Check sheet for the drawn part. Datum: minimum x, y, z corner. Units: mm. Give positions to 0.01 mm unless a question says otherwise; leave off trailing zeros. Order: outer loops, then holes, each group sorted by start corner. A loop starts at its lowest first (then second) coordinate and runs counter-clockwise, first axis right, second up.
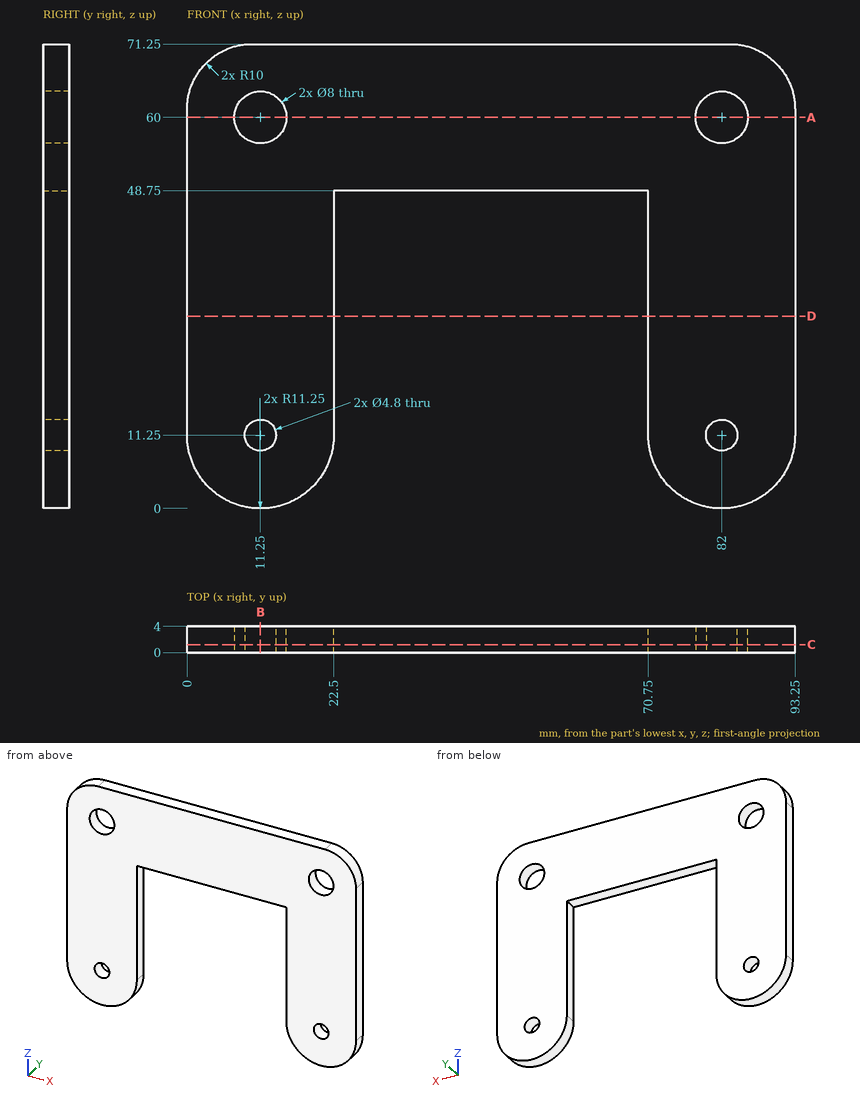
Item 1: Scan lines: L1, parallel to X at y = 3.15, z = 60; L2, parallel to Z at x = 82, y = 3.1; L3, parallel to X at y = 3.25, z = 24.5. Record each from-to range of solid material in increasing order.
Reported:
L1: x = 0 to 7.25, 15.25 to 78, 86 to 93.25
L2: z = 0 to 8.85, 13.65 to 56, 64 to 71.25
L3: x = 0 to 22.5, 70.75 to 93.25
Item 2: Sectioned sample at C-C (y = 1.2). Enter the section's corners in (x, z).
Reported:
outline: (0, 11.25) arc R11.25 ccw to (22.5, 11.25) - (22.5, 48.75) - (70.75, 48.75) - (70.75, 11.25) arc R11.25 ccw to (93.25, 11.25) - (93.25, 61.25) arc R10 ccw to (83.25, 71.25) - (10, 71.25) arc R10 ccw to (0, 61.25) - close; hole circle Ø8 at (11.25, 60); hole circle Ø4.8 at (11.25, 11.25); hole circle Ø8 at (82, 60); hole circle Ø4.8 at (82, 11.25)
Item 3: Sectioned sample at A-A (z = 60). Enter the section's corners in (x, y), and give its area (3 significant figures).
Reported:
outline: (0, 0) - (7.25, 0) - (7.25, 4) - (0, 4) - close; (15.25, 0) - (78, 0) - (78, 4) - (15.25, 4) - close; (86, 0) - (93.25, 0) - (93.25, 4) - (86, 4) - close
area: 309 mm2
Item 4: Gauge pin test, flat end, axial feed: pin 1 (2 mm diameter, centred on x = 47.5, y = 2, fed in from -Z). Record the tip position at first contact, or that the pin passes through.
Reported:
pin 1: stops at z = 48.75
Item 5: Sectioned sample at D-D (z = 29.5). Enter the section's corners in (x, y), and give its area (3 significant figures).
Reported:
outline: (0, 0) - (22.5, 0) - (22.5, 4) - (0, 4) - close; (70.75, 0) - (93.25, 0) - (93.25, 4) - (70.75, 4) - close
area: 180 mm2
Item 6: Sectioned sample at B-B (x = 11.25). Enter the section's corners in (y, z), and give its area (3 significant figures).
Reported:
outline: (0, 0) - (4, 0) - (4, 8.85) - (0, 8.85) - close; (0, 13.65) - (4, 13.65) - (4, 56) - (0, 56) - close; (0, 64) - (4, 64) - (4, 71.25) - (0, 71.25) - close
area: 234 mm2
